Input: dimensioned drawing with shaded views. Units: mm. Origin: part minimum x, y, z. Coordinates: 2 decimals unless noted, no trailing zeros. Order: outer loops, then holes, each group sorted by start corner. A loop starts at its lowest first (then second) coordinate and runs counter-clockwise, first axis right, second up. Notation, with made-up numbers: M -4.5,-28 L 10.5,-28 A24 cw 10.5,7 Z; hole C 70.5,-9.5 d8. An arc over 180 degrees is marked long. Write item = value, one per line.
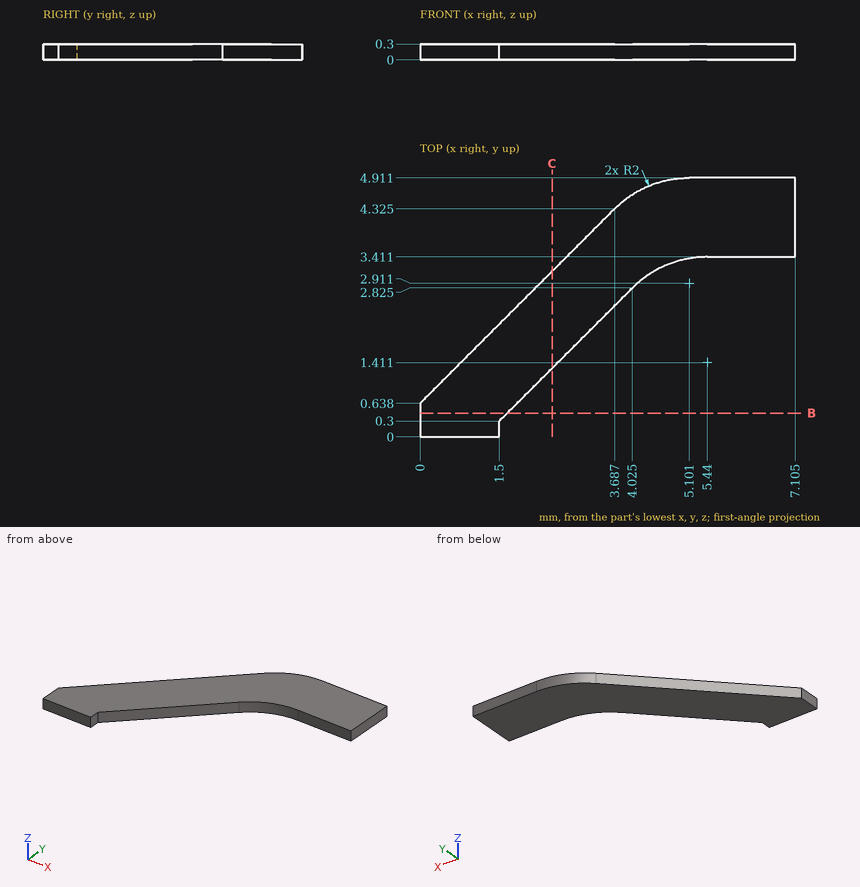
1) Section B-B, the plane y = 0.45. Return loops of the section in (x, z).
Numbers:
outline = M 0,0 L 1.65,0 L 1.65,0.3 L 0,0.3 Z
2) Section C-C, the plane x = 2.5. Return loops of the section in (y, z).
Numbers:
outline = M 1.3,0 L 3.14,0 L 3.14,0.3 L 1.3,0.3 Z
3) Line query: L1, parallel to Y at x = 6, z = 0.1; L2, parallel to X at y = 0.2, z = 0.1; L3, parallel to Y at x = 2, z = 0.2. Output: solid intervals per line, ascending.
Numbers:
L1 = 3.41 to 4.91
L2 = 0 to 1.5
L3 = 0.8 to 2.64
